For this review, take the finished solid that the model builds, in its own axes (mm). Face numbers are marked on the shaded views. A direction names the side the tool comes from. Round coordinates to 2 decimals unless told otherwise and drop trailing zeros. Order: outer loops, then holes, each group sorted by start corner. A loop starts at its lowest first (then second) coordinate and runs counter-clockwise, first axis right, second up. Notation, with made-up numbers: M 60,13.25 L 78,13.25 A25 ccw 78,40.25 Z; hole C -21,-32.75 d7. An arc over 180 degrees is marked long. Answer as a JSON object with one key per item and string values.
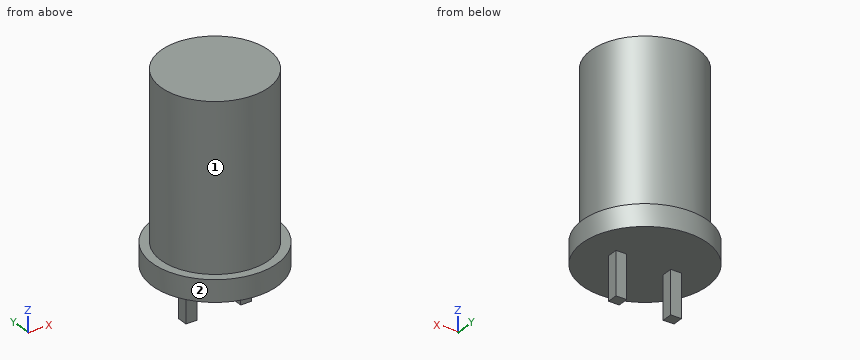
from build123d import *

# Parameters (mm, degrees)
BODY_START   = -8.6
SKETCH1_R    = 2.5
BODY_DEPTH   = 8.6
FLANGE_START = -8.6
SKETCH2_R    = 2.9
FLANGE_DEPTH = 1
LEADS_START  = -8.6
SKETCH3_W    = 0.5
SKETCH3_H    = 0.5
LEADS_DEPTH  = 2


with BuildPart() as part:
    # Sketch1 → Body (new body)
    with BuildSketch(Plane.XY.offset(BODY_START)):
        with Locations(Location((0, 0, 0), (0, 0, 180))):
            Circle(SKETCH1_R)
    extrude(amount=BODY_DEPTH)

    # Sketch2 → Flange (add)
    with BuildSketch(Plane.XY.offset(FLANGE_START)):
        Circle(SKETCH2_R)
    extrude(amount=FLANGE_DEPTH)

    # Sketch3 → Leads (add)
    with BuildSketch(Plane.XY.offset(LEADS_START)):
        with Locations((-1.27, 0)):
            Rectangle(SKETCH3_W, SKETCH3_H)
        with Locations((1.27, 0)):
            Rectangle(SKETCH3_W, SKETCH3_H)
    extrude(amount=-LEADS_DEPTH)


solid = part.part
1) Add section A-A on z = -9.5. State the section outline as (x, y) points.
Geometry check:
{"outline": "M -1.52,-0.25 L -1.02,-0.25 L -1.02,0.25 L -1.52,0.25 Z; M 1.02,-0.25 L 1.52,-0.25 L 1.52,0.25 L 1.02,0.25 Z"}
2) Add section C-C on y = 0. State the section outline as (x, z) points.
Geometry check:
{"outline": "M -2.9,-8.6 L -1.52,-8.6 L -1.52,-10.6 L -1.02,-10.6 L -1.02,-8.6 L 1.02,-8.6 L 1.02,-10.6 L 1.52,-10.6 L 1.52,-8.6 L 2.9,-8.6 L 2.9,-7.6 L 2.5,-7.6 L 2.5,0 L -2.5,0 L -2.5,-7.6 L -2.9,-7.6 Z"}
3) Machinability: for the marked faces 1 and 2, which of the approach directions +Z, -Z, +X, -X, +Y, -Y give a long, thin tool a straight path to every point of the face, cutting with its end or side? Answer none if there is none.
Geometry check:
{"face 1": "+Z", "face 2": "+Z, -Z"}
4) For L1, parallel to Z at x = 1, y = 0.5; L2, parallel to Z at x = 1.1, y = -2.5; L3, parallel to X at y = 0.1, z = -2.75, list the stretches that pass through material, from the lowest coordinate up.
Geometry check:
{"L1": "z = -8.6 to 0", "L2": "z = -8.6 to -7.6", "L3": "x = -2.5 to 2.5"}
5) Insertion check: P1, Ø0.6, axis at y = 0, z = -10, coming from the -X side; P2, Ø1.5, axis at x = 1, z = -1.5, coming from the -Y side. Each pin has a flat end and moves straight along its axis. Give the tip position at first contact, or say it passes through.
Geometry check:
{"P1": "stops at x = -1.52", "P2": "stops at y = -2.49"}
6) Add section D-D on z = -5.25. State the section outline as (x, y) points.
Geometry check:
{"outline": "C 0,0 d5"}
7) Add section B-B on x = 0. State the section outline as (y, z) points.
Geometry check:
{"outline": "M -2.9,-8.6 L 2.9,-8.6 L 2.9,-7.6 L 2.5,-7.6 L 2.5,0 L -2.5,0 L -2.5,-7.6 L -2.9,-7.6 Z"}
